Geometry check sheet. Reference: the model listing, model coordinates, mm. Face numbers are marked on the shaded views. Round coordinates to 2 decimals unless told otherwise and drop trailing zeros. Write each loop counter-clockwise with the first axis right and the second up, starting at its lowest first coordinate (ties: lowest second). Pieces come first, ordered by that corner, then holes. Notation, with made-up numbers: (82.25, 7) -> (130.25, 7) arc R17 ccw to (130.25, 23) -> close; hole circle Ø8 at (19, 42). An arc over 180 degrees is marked (long way). One line per question, with ' | ' between items.
```python
from build123d import *

# Parameters (mm, degrees)
SKETCH2_W           = 50
SKETCH2_H           = 200
BOSS_EXTRUDE2_DEPTH = 10
SKETCH4_R           = 6
BOSS_EXTRUDE3_DEPTH = 7
SKETCH5_R           = 7.5
BOSS_EXTRUDE4_DEPTH = 2
SKETCH8_W           = 20.1
SKETCH8_H           = 20.1
CUT_EXTRUDE4_DEPTH  = 3
SKETCH9_R           = 1.6
CUT_EXTRUDE5_DEPTH  = 129.570250184
CUT_EXTRUDE8_REACH  = 131.411
SKETCH10_W          = 20
SKETCH10_H          = 23.413423022
SKETCH10_H_2        = 20.071314626
SKETCH11_R          = 4.05
CUT_EXTRUDE9_DEPTH  = 9
SKETCH12_R          = 1.6
CUT_EXTRUDE10_DEPTH = 129.399023487
FILLET2_R           = 2
FILLET3_R           = 1
CHAMFER1_SIZE       = 3
SKETCH14_R          = 1.65
CUT_EXTRUDE12_DEPTH = 130.411395296
SKETCH15_W          = 3.1
SKETCH15_H          = 10.1
CUT_EXTRUDE13_DEPTH = 206.006939607
SKETCH16_W          = 22.2
SKETCH16_H          = 10
CUT_EXTRUDE14_DEPTH = 10
SKETCH17_R          = 1.6
CUT_EXTRUDE15_DEPTH = 130.411395296
SKETCH18_R          = 1.6
CUT_EXTRUDE16_DEPTH = 129.570250184
SKETCH19_R          = 1.6
CUT_EXTRUDE17_DEPTH = 129.570250184


with BuildPart() as part:
    # Sketch2 → Boss-Extrude2 (new body)
    with BuildSketch(Plane(origin=(0, 0, 0), x_dir=(0, 0, -1), z_dir=(1, 0, 0))):
        with Locations((-15.827016632, 21.323797935)):
            Rectangle(SKETCH2_W, SKETCH2_H)
    extrude(amount=BOSS_EXTRUDE2_DEPTH)

    # Sketch4 → Boss-Extrude3 (add)
    with BuildSketch(Plane(origin=(10, 0, 0), x_dir=(0, 0, -1), z_dir=(1, 0, 0))):
        with Locations((-20.827016632, 106.323797935)):
            Circle(SKETCH4_R)
        with Locations((-20.827016632, -63.676202065)):
            Circle(SKETCH4_R)
    extrude(amount=BOSS_EXTRUDE3_DEPTH)

    # Sketch5 → Boss-Extrude4 (add)
    with BuildSketch(Plane(origin=(17, 0, 0), x_dir=(0, 0, -1), z_dir=(1, 0, 0))):
        with Locations((-20.827016632, -63.676202065)):
            Circle(SKETCH5_R)
        with Locations((-20.827016632, 106.323797935)):
            Circle(SKETCH5_R)
    extrude(amount=BOSS_EXTRUDE4_DEPTH)

    # Sketch8 → Cut-Extrude4 (cut)
    with BuildSketch(Plane(origin=(10, 0, 0), x_dir=(0, 0, -1), z_dir=(1, 0, 0))):
        with Locations((-0.877016632, -68.626202065)):
            Rectangle(SKETCH8_W, SKETCH8_H)
        with Locations((-0.877016632, 111.273797935)):
            Rectangle(SKETCH8_W, SKETCH8_H)
    extrude(amount=-CUT_EXTRUDE4_DEPTH, mode=Mode.SUBTRACT)

    # Sketch9 → Cut-Extrude5 (cut, through all)
    with BuildSketch(Plane(origin=(7, 0, 0), x_dir=(0, 0, -1), z_dir=(1, 0, 0))):
        with Locations((-5.827016632, 114.323797935)):
            Circle(SKETCH9_R)
        with Locations((2.172983368, 105.323797935)):
            Circle(SKETCH9_R)
        with Locations((2.172983368, 114.323797935)):
            Circle(SKETCH9_R)
        with Locations((-5.827016632, -71.676202065)):
            Circle(SKETCH9_R)
        with Locations((2.172983368, -62.676202065)):
            Circle(SKETCH9_R)
        with Locations((2.172983368, -71.676202065)):
            Circle(SKETCH9_R)
    extrude(amount=-CUT_EXTRUDE5_DEPTH, mode=Mode.SUBTRACT)

    # Cut-Extrude8: up to this face of the body (flat: up to its plane)
    cut_extrude8_end = Plane(part.part.faces().sort_by_distance((10, 21.323797935, 17.048206438))[0])
    # Sketch10 → Cut-Extrude8 (cut, up to the picked face)
    with BuildSketch(Plane(origin=(19, 0, 0), x_dir=(0, 0, -1), z_dir=(1, 0, 0)), mode=Mode.PRIVATE) as cut_extrude8_sk1:
        with Locations((-30.827016632, -63.1074113)):
            Rectangle(SKETCH10_W, SKETCH10_H)
    cut_extrude8_tool1 = split(extrude(cut_extrude8_sk1.sketch, amount=-CUT_EXTRUDE8_REACH, mode=Mode.PRIVATE), bisect_by=cut_extrude8_end, keep=Keep.BOTH, mode=Mode.PRIVATE)
    # Sketch10 → Cut-Extrude8 (cut, up to the picked face)
    with BuildSketch(Plane(origin=(19, 0, 0), x_dir=(0, 0, -1), z_dir=(1, 0, 0)), mode=Mode.PRIVATE) as cut_extrude8_sk2:
        with Locations((-30.827016632, 105.037131871)):
            Rectangle(SKETCH10_W, SKETCH10_H_2)
    cut_extrude8_tool2 = split(extrude(cut_extrude8_sk2.sketch, amount=-CUT_EXTRUDE8_REACH, mode=Mode.PRIVATE), bisect_by=cut_extrude8_end, keep=Keep.BOTH, mode=Mode.PRIVATE)
    add(cut_extrude8_tool1.solids().sort_by(Axis((19, -63.107411, 30.827017), (-1, 0, 0)))[0], mode=Mode.SUBTRACT)
    add(cut_extrude8_tool2.solids().sort_by(Axis((19, 105.037132, 30.827017), (-1, 0, 0)))[0], mode=Mode.SUBTRACT)

    # Sketch11 → Cut-Extrude9 (cut)
    with BuildSketch(Plane(origin=(19, 0, 0), x_dir=(0, 0, -1), z_dir=(1, 0, 0))):
        with Locations((-20.827016632, -63.676202065)):
            Circle(SKETCH11_R)
        with Locations((-20.827016632, 106.323797935)):
            Circle(SKETCH11_R)
    extrude(amount=-CUT_EXTRUDE9_DEPTH, mode=Mode.SUBTRACT)

    # Sketch12 → Cut-Extrude10 (cut, through all)
    with BuildSketch(Plane(origin=(10, 0, 0), x_dir=(0, 0, -1), z_dir=(1, 0, 0))):
        with Locations((-23.027016632, 39.323797935)):
            Circle(SKETCH12_R)
        with Locations((-23.027016632, 88.323797935)):
            Circle(SKETCH12_R)
        with Locations((-0.827016632, 88.323797935)):
            Circle(SKETCH12_R)
        with Locations((-0.827016632, 39.323797935)):
            Circle(SKETCH12_R)
    extrude(amount=-CUT_EXTRUDE10_DEPTH, mode=Mode.SUBTRACT)

    # Fillet2
    # the kernel refuses this fillet: 2 mm, written as the material it adds along each edge
    with BuildSketch(Plane(origin=(17, 106.323797935, 20.827016632), x_dir=(0, 1, 0), z_dir=(0, 0, 1))) as fillet2_piece_1:
        with BuildLine():
            CenterArc((8, 1.936491673), FILLET2_R, 180, 75.522487814)
            Line((7.5, 0), (7.49, -0.038729833))
            ThreePointArc((7.49, -0.038729833), (6.75, -0.04), (6, -0.04))
            Line((6, -0.04), (5.96, 0))
            Line((5.96, 0), (5.96, 1.936491673))
            Line((5.96, 1.936491673), (6, 1.936491673))
        make_face()
    revolve(axis=Axis((17, 106.323797935, 20.827016632), (-1, 0, 0)), revolution_arc=180)
    with BuildSketch(Plane(origin=(17, -63.676202065, 20.827016632), x_dir=(0, -1, 0), z_dir=(0, 0, 1))) as fillet2_piece_2:
        with BuildLine():
            CenterArc((8, -1.936491673), FILLET2_R, 104.477512186, 75.522487814)
            Line((6, -1.936491673), (5.96, -1.936491673))
            Line((5.96, -1.936491673), (5.96, 0))
            Line((5.96, 0), (6, 0.04))
            ThreePointArc((6, 0.04), (6.75, 0.04), (7.49, 0.038729833))
            Line((7.49, 0.038729833), (7.5, 0))
        make_face()
    revolve(axis=Axis((17, -63.676202065, 20.827016632), (1, 0, 0)), revolution_arc=180)

    # Fillet3
    fillet3_edges = [part.edges().sort_by_distance(p)[0] for p in [
        (0, 121.323797935, 15.827016632),
        (0, 21.323797935, -9.172983368),
        (0, -78.676202065, 15.827016632),
        (0, 21.323797935, 40.827016632),
    ]]
    fillet(fillet3_edges, radius=FILLET3_R)

    # Chamfer1
    chamfer1_edges = [part.edges().sort_by_distance(p)[0] for p in [
        (10, -63.676202065, 14.827016632),
        (10, 106.323797935, 14.827016632),
    ]]
    chamfer(chamfer1_edges, length=CHAMFER1_SIZE)

    # Sketch14 → Cut-Extrude12 (cut, through all)
    with BuildSketch(Plane.ZY):
        with Locations((34.827016632, 111.323797935)):
            Circle(SKETCH14_R)
        with Locations((34.827016632, 66.323797935)):
            Circle(SKETCH14_R)
        with Locations((34.827016632, 21.323797935)):
            Circle(SKETCH14_R)
        with Locations((34.827016632, -23.676202065)):
            Circle(SKETCH14_R)
        with Locations((34.827016632, -68.676202065)):
            Circle(SKETCH14_R)
    extrude(amount=-CUT_EXTRUDE12_DEPTH, mode=Mode.SUBTRACT)

    # Sketch15 → Cut-Extrude13 (cut, through all)
    with BuildSketch(Plane.XZ.offset(78.676202065)):
        with Locations((8.45, 35.777016632)):
            Rectangle(SKETCH15_W, SKETCH15_H)
    extrude(amount=-CUT_EXTRUDE13_DEPTH, mode=Mode.SUBTRACT)

    # Sketch16 → Cut-Extrude14 (cut)
    with BuildSketch(Plane(origin=(10, 0, 0), x_dir=(0, 0, -1), z_dir=(1, 0, 0))):
        with Locations((-11.927016632, 5.273797935)):
            Rectangle(SKETCH16_W, SKETCH16_H)
    extrude(amount=-CUT_EXTRUDE14_DEPTH, mode=Mode.SUBTRACT)

    # Sketch17 → Cut-Extrude15 (cut, through all)
    with BuildSketch(Plane.ZY):
        with Locations((26.027016632, 5.273797935)):
            Circle(SKETCH17_R)
        with Locations((-2.172983368, 5.273797935)):
            Circle(SKETCH17_R)
    extrude(amount=-CUT_EXTRUDE15_DEPTH, mode=Mode.SUBTRACT)

    # Sketch18 → Cut-Extrude16 (cut, through all)
    with BuildSketch(Plane(origin=(7, 0, 0), x_dir=(0, 0, -1), z_dir=(1, 0, 0))):
        with Locations((-5.827016632, -62.676202065)):
            Circle(SKETCH18_R)
    extrude(amount=-CUT_EXTRUDE16_DEPTH, mode=Mode.SUBTRACT)

    # Sketch19 → Cut-Extrude17 (cut, through all)
    with BuildSketch(Plane(origin=(7, 0, 0), x_dir=(0, 0, -1), z_dir=(1, 0, 0))):
        with Locations((-5.827016632, 105.323797935)):
            Circle(SKETCH19_R)
    extrude(amount=-CUT_EXTRUDE17_DEPTH, mode=Mode.SUBTRACT)


solid = part.part
```
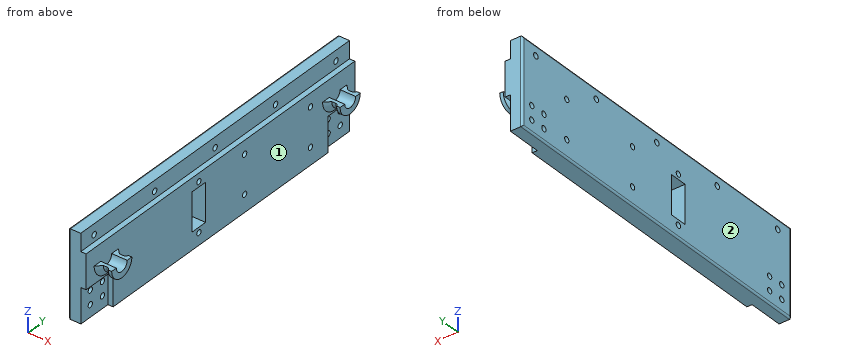
(1) Go/stop test with flat-tipped pins: pin 1 (5 mm diameter, centred on y = 105.32, z = 5.83, fed in from +X); pin 2 (2 mm diameter, centred on x = 10.5, y = 41.5, fed in from +Z); pin 3 (3 mm diameter, centred on y = 114.32, z = 5.83, fed in from +X); pin 4 (4 mm diameter, centred on y = 39.32, z = 23.03, fed in from +X). Record where each tip stops, or that it passes through.
Resolved:
pin 1: stops at x = 7 | pin 2: stops at z = 30.73 | pin 3: passes through | pin 4: stops at x = 10
(2) Sectioned sample at A-A on y = 53. Record the cut outline in (x, z), then the cut area to 3 significant figures.
Resolved:
outline: (0, -8.17) arc R1 ccw to (1, -9.17) -> (10, -9.17) -> (10, 30.73) -> (6.9, 30.73) -> (6.9, 40.83) -> (1, 40.83) arc R1 ccw to (0, 39.83) -> close | area: 468 mm2
(3) Sectioned sample at B-B on x = 5. Count the separate pieces of the cut face and the enclosed holes in it, then the cut area to 3 significant figures.
Resolved:
separate pieces: 1 | enclosed holes: 20 | area: 9,620 mm2
(4) Material ranges on line 1 (Z direction, x = 6.25, y = 10); line 2 (Y direction, x = 2.75, z = 24); line 3 (X direction, y = 2, z = -5.5), recorded low to high.
Resolved:
line 1: z = -9.17 to 0.83, 23.03 to 40.83 | line 2: y = -78.68 to 38.05, 40.59 to 87.05, 89.59 to 121.32 | line 3: x = 0 to 10
(5) Draft check along Y on the marked faces 1 and 2. Enter one of: +Y half, -Y half, draft (parallel to the pull), parting line (faces both ways), or undercut.
Resolved:
face 1: undercut | face 2: draft
